Input: part model. Units: mm. Frame: model coordinates. A direction names the side the tool comes from. Round coordinates to 2 decimals unless told otherwise and drop trailing zeros. Loops run counter-clockwise (first coordinate to the right, second up) from the corner with the lowest first, then second, coordinate; pieces in that order, holes last.
1) First-contact query: pin 1 (8 mm diameter, centred on x = 40.5, z = 7, fed in from +Y); pin 2 (8.5 mm diameter, centred on x = 43.5, z = 19, fed in from -Y); pin 3 (5.5 mm diameter, centred on x = 7.5, z = 8.5, fed in from +Y). Flat tips, straight axial feed; report the tip coordinate or a pass-through.
2) Section A-A, the plane y = 14.5. Return loops of the section in (x, z).
3) Section B-B, the plane x = 55.88. Return loops of the section in (y, z), and give its area (3 significant figures).
4) Access query for faces 1 (the face through (0.362, 9.641, 0.382)), 2 (the face through (1.321, 9, 16)), 3 (the face through (24, 19.05, 8)). Directions: +Z, -Z, +X, -X, +Y, -Y. A direction counts if a zero-diameter tool reaches every point of the face in a straight line with its end or side. Return the directions, or none.
5) Ray query, line 1 along Z through (x, y) = (32, 5.5); line 2 along X through (y, z) = (9, 30); line 3 along Y through (x, z) = (53.5, 12). Return the intervals inside material, ascending.
6) Section D-D, the plane x = 14. Return loops of the section in (y, z).
7) Draft query along Z for faces 4 (the face through (31, 10, 31.75)), 5 (the face through (5.96, 21.55, 10.87)), 6 (the face through (0.362, 0.382, 16.079)). Return one class per face: pulls with the +Z half, pulls with the -Z half, needs draft (parallel to the pull), parting line crosses it, or undercut.
8) Section C-C, the plane y = 22.25. State how many separate pieces and enclosed holes the cut face has, and give its area (3 significant figures).
from build123d import *

# Parameters (mm, degrees)
F0_W     = 63.5
F0_H     = 19.05
F1_DEPTH = 31.75
F2_T     = -1.3208
F3_R     = 4.6736
F3_R_2   = 3.556
F4_DEPTH = 5.08
F5_R     = 1.27


with BuildPart() as f1:
    # F0 (on Top) → F1 (new body)
    with BuildSketch(Plane.XY):
        with Locations((31.75, 9.525)):
            Rectangle(F0_W, F0_H)
    extrude(amount=F1_DEPTH)

    # F2
    f2_openings = [f1.faces().sort_by_distance(p)[0] for p in [
        (31.75, 0, 15.875),
    ]]
    offset(amount=F2_T, openings=f2_openings)

    # F3 (on face) → F4 (join)
    with BuildSketch(Plane(origin=(0, 19.05, 0), x_dir=(-1, 0, 0), z_dir=(0, 1, 0))):
        with Locations((-7.874, 23.876)):
            Circle(F3_R)
        with Locations((-7.874, 23.876)):
            Circle(F3_R_2, mode=Mode.SUBTRACT)
        with Locations((-23.876, 23.876)):
            Circle(F3_R)
        with Locations((-23.876, 23.876)):
            Circle(F3_R_2, mode=Mode.SUBTRACT)
        with Locations((-39.878, 23.876)):
            Circle(F3_R)
        with Locations((-39.878, 23.876)):
            Circle(F3_R_2, mode=Mode.SUBTRACT)
        with Locations((-55.88, 23.876)):
            Circle(F3_R)
        with Locations((-55.88, 23.876)):
            Circle(F3_R_2, mode=Mode.SUBTRACT)
        with Locations((-55.88, 7.874)):
            Circle(F3_R)
        with Locations((-55.88, 7.874)):
            Circle(F3_R_2, mode=Mode.SUBTRACT)
        with Locations((-39.878, 7.874)):
            Circle(F3_R)
        with Locations((-39.878, 7.874)):
            Circle(F3_R_2, mode=Mode.SUBTRACT)
        with Locations((-23.876, 7.874)):
            Circle(F3_R)
        with Locations((-23.876, 7.874)):
            Circle(F3_R_2, mode=Mode.SUBTRACT)
        with Locations((-7.874, 7.874)):
            Circle(F3_R)
        with Locations((-7.874, 7.874)):
            Circle(F3_R_2, mode=Mode.SUBTRACT)
    extrude(amount=F4_DEPTH)

    # F5
    f5_edges = [f1.edges().sort_by_distance(p)[0] for p in [
        (0, 9.525, 31.75),
        (31.75, 0, 31.75),
        (63.5, 9.525, 31.75),
        (31.75, 19.05, 31.75),
        (0, 19.05, 15.875),
        (0, 0, 15.875),
        (0, 9.525, 0),
        (31.75, 0, 0),
        (63.5, 9.525, 0),
        (31.75, 19.05, 0),
        (63.5, 0, 15.875),
        (63.5, 19.05, 15.875),
    ]]
    fillet(f5_edges, radius=F5_R)


solid = f1.part
Final values:
1. pin 1: stops at y = 24.13
1. pin 2: stops at y = 17.73
1. pin 3: stops at y = 19.05
2. outline: (0, 1.27) arc R1.27 ccw to (1.27, 0) - (62.23, 0) arc R1.27 ccw to (63.5, 1.27) - (63.5, 30.48) arc R1.27 ccw to (62.23, 31.75) - (1.27, 31.75) arc R1.27 ccw to (0, 30.48) - close; hole (1.32, 1.32) - (62.18, 1.32) - (62.18, 30.43) - (1.32, 30.43) - close
3. outline: (0, 1.27) arc R1.27 ccw to (1.27, 0) - (17.78, 0) arc R1.27 ccw to (19.05, 1.27) - (19.05, 3.2) - (24.13, 3.2) - (24.13, 4.32) - (19.05, 4.32) - (19.05, 11.43) - (24.13, 11.43) - (24.13, 12.55) - (19.05, 12.55) - (19.05, 19.2) - (24.13, 19.2) - (24.13, 20.32) - (19.05, 20.32) - (19.05, 27.43) - (24.13, 27.43) - (24.13, 28.55) - (19.05, 28.55) - (19.05, 30.48) arc R1.27 ccw to (17.78, 31.75) - (1.27, 31.75) arc R1.27 ccw to (0, 30.48) - (0, 30.43) - (17.73, 30.43) - (17.73, 1.32) - (0, 1.32) - close
3. area: 110 mm2
4. face 1: -Z, -X, +Y, -Y
4. face 2: -Y
4. face 3: +Y
5. line 1: z = 0 to 1.32, 30.43 to 31.75
5. line 2: x = 0 to 1.32, 62.18 to 63.5
5. line 3: y = 17.73 to 19.05
6. outline: (0, 1.27) arc R1.27 ccw to (1.27, 0) - (17.78, 0) arc R1.27 ccw to (19.05, 1.27) - (19.05, 30.48) arc R1.27 ccw to (17.78, 31.75) - (1.27, 31.75) arc R1.27 ccw to (0, 30.48) - (0, 30.43) - (17.73, 30.43) - (17.73, 1.32) - (0, 1.32) - close
7. face 4: pulls with the +Z half
7. face 5: undercut
7. face 6: needs draft
8. separate pieces: 8
8. enclosed holes: 8
8. area: 231 mm2
